Work out the finished part from the listing and answer in its coordinate system (mm). Face numbers are marked on the shaded views. A direction names the side the tool comes from. Give positions to 0.01 mm unless a question says otherwise; leave off trailing zeros. Order: outer loops, then holes, each group sorted by start corner. A loop starts at its lowest first (then second) coordinate and runs counter-clockwise, first axis right, second up.
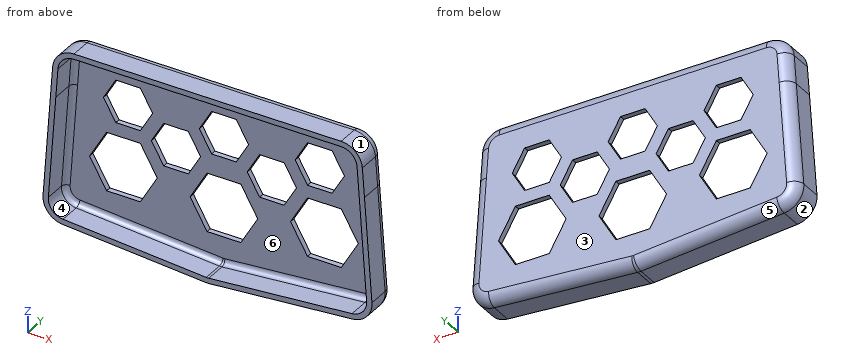
```python
from build123d import *

# Parameters (mm, degrees)
BOSS_EXTRUDE1_DEPTH     = 38.1
FILLET1_R               = 25.4
FILLET2_R               = 12.7
SHELL1_T                = -6.35
CUT_EXTRUDE1_DEPTH      = 255.858427337
CUT_EXTRUDE1_DEPTH_BACK = 255.858427337


with BuildPart() as part:
    # Sketch1 → Boss-Extrude1 (new body)
    with BuildSketch(Plane(origin=(0, 0, 0), x_dir=(1, 0, 0), z_dir=(0, 1, 0))):
        Polygon((-114.3, -63.5), (114.3, -63.5), (182.894154879, -63.5), (187.132137575, -5.303806299), (197.900067, 142.561947658), (0, 158.296586732), (-197.900067, 142.561947658), (-187.132137575, -5.303806299), (-182.894154879, -63.5), align=None)
    extrude(amount=BOSS_EXTRUDE1_DEPTH)

    # Fillet1
    fillet1_edges = [part.edges().sort_by_distance(p)[0] for p in [
        (-182.894154879, 19.05, 63.5),
        (-197.900067, 19.05, -142.561947658),
        (0, 19.05, -158.296586732),
        (197.900067, 19.05, -142.561947658),
        (182.894154879, 19.05, 63.5),
    ]]
    fillet(fillet1_edges, radius=FILLET1_R)

    # Fillet2
    fillet2_edges = [part.edges().sort_by_distance(p)[0] for p in [
        (190.338493083, 38.1, -38.72603044),
        (0, 38.1, 63.5),
        (87.380434893, 38.1, -151.349142873),
        (-87.380434893, 38.1, -151.349142873),
        (-190.338493083, 38.1, -38.72603044),
        (-190.007212355, 38.1, -135.786308877),
        (0, 38.1, -158.216429875),
        (-176.572564505, 38.1, 56.70131683),
        (190.007212355, 38.1, -135.786308877),
        (176.572564505, 38.1, 56.70131683),
    ]]
    fillet(fillet2_edges, radius=FILLET2_R)

    # Shell1
    shell1_openings = [part.faces().sort_by_distance(p)[0] for p in [
        (0, 0, -44.95160626),
    ]]
    offset(amount=SHELL1_T, openings=shell1_openings, kind=Kind.INTERSECTION)

    # Sketch3 → Cut-Extrude1 (cut, two sides: drawn at the far end of the back side and taken through both)
    with BuildSketch(Plane(origin=(0, 38.1, 0), x_dir=(1, 0, 0), z_dir=(0, 1, 0)).offset(-CUT_EXTRUDE1_DEPTH_BACK)):
        Polygon((-128.964696837, 25.4), (-143.629393675, 0), (-128.964696837, -25.4), (-99.635303163, -25.4), (-84.970606325, 0), (-99.635303163, 25.4), align=None)
        Polygon((-27.820606325, 32.995567884), (-42.485303163, 58.395567884), (-71.814696837, 58.395567884), (-86.479393675, 32.995567884), (-71.814696837, 7.595567884), (-42.485303163, 7.595567884), align=None)
        Polygon((40.327916303, 85.041135768), (20.163958151, 119.966135768), (-20.163958151, 119.966135768), (-40.327916303, 85.041135768), (-20.163958151, 50.116135768), (20.163958151, 50.116135768), align=None)
        Polygon((29.329393675, 0), (14.664696837, 25.4), (-14.664696837, 25.4), (-29.329393675, 0), (-14.664696837, -25.4), (14.664696837, -25.4), align=None)
        Polygon((143.629393675, 0), (128.964696837, 25.4), (99.635303163, 25.4), (84.970606325, 0), (99.635303163, -25.4), (128.964696837, -25.4), align=None)
        Polygon((71.814696837, 7.595567884), (86.479393675, 32.995567884), (71.814696837, 58.395567884), (42.485303163, 58.395567884), (27.820606325, 32.995567884), (42.485303163, 7.595567884), align=None)
        Polygon((-99.635303163, 40.591135768), (-79.471345011, 75.516135768), (-99.635303163, 110.441135768), (-139.963219465, 110.441135768), (-160.127177617, 75.516135768), (-139.963219465, 40.591135768), align=None)
        Polygon((160.127177617, 75.516135768), (139.963219465, 110.441135768), (99.635303163, 110.441135768), (79.471345011, 75.516135768), (99.635303163, 40.591135768), (139.963219465, 40.591135768), align=None)
    extrude(amount=CUT_EXTRUDE1_DEPTH + CUT_EXTRUDE1_DEPTH_BACK, mode=Mode.SUBTRACT)


solid = part.part
```
1. The part is cut by section A-A (y = 6.5). Write down the section's boundary in (x, z).
Findings below:
outline: (-196.07, -117.4) arc R25.4 ccw to (-172.75, -144.56) - (-2.01, -158.14) arc R25.4 ccw to (2.01, -158.14) - (172.75, -144.56) arc R25.4 ccw to (196.07, -117.4) - (184.61, 39.94) arc R25.4 ccw to (159.28, 63.5) - (-159.28, 63.5) arc R25.4 ccw to (-184.61, 39.94) - close; hole (-189.73, -117.86) arc R19.05 ccw to (-172.24, -138.23) - (-1.51, -151.81) arc R19.05 ccw to (1.51, -151.81) - (172.24, -138.23) arc R19.05 ccw to (189.73, -117.86) - (178.28, 39.48) arc R19.05 ccw to (159.28, 57.15) - (-159.28, 57.15) arc R19.05 ccw to (-178.28, 39.48) - close
2. The part is cut by section B-B (x = -110.5). State how many separate pieces and enclosed holes the cut face has, then the cut area to 3 significant figures.
Findings below:
separate pieces: 3
enclosed holes: 0
area: 938 mm2
3. The mould has two halves that part along X. Classify the marked faces 1, 2, 3 and 4: pulls with the +X half, pulls with the -X half, needs draft (parallel to the pull), parting line crosses it, or undercut.
Findings below:
face 1: pulls with the +X half
face 2: pulls with the -X half
face 3: needs draft
face 4: undercut
4. Given P1, Ø1.5, axis at x = -140.5, z = -19, coming from the -Y side; P2, Ø1.9, axis at x = 111.5, y = 35, coming from the -Z side; P3, Ø3, axis at x = -55, y = 34.5, coming from the -Z side, each flat-ended and moving along its own axis, determine where each tip first touches the part or whether it passes through.
Findings below:
P1: stops at y = 31.75
P2: stops at z = -146.02
P3: stops at z = -151.4
5. Which of the six approach directions +Z, -Z, +X, -X, +Y, -Y give full straight-line access (tool end or side, diameter ignored) to the marked faces 5 and 6?
Findings below:
face 5: -Z, -X, +Y
face 6: -Y
6. Straight lines are drawn through the part: probe 1 along Z at (x, y) = (-109, 32.5); probe 2 along Y at (x, z) = (-162.5, -88.5); probe 3 along X at (y, z) = (33, -110). For each, find the intervals that lie inside material, in ascending order.
Findings below:
probe 1: z = -147.45 to -110.44, -40.59 to -25.4, 25.4 to 61.33
probe 2: y = 31.75 to 38.1
probe 3: x = -193 to -140.22, -99.38 to -25.92, 25.92 to 99.38, 140.22 to 193
